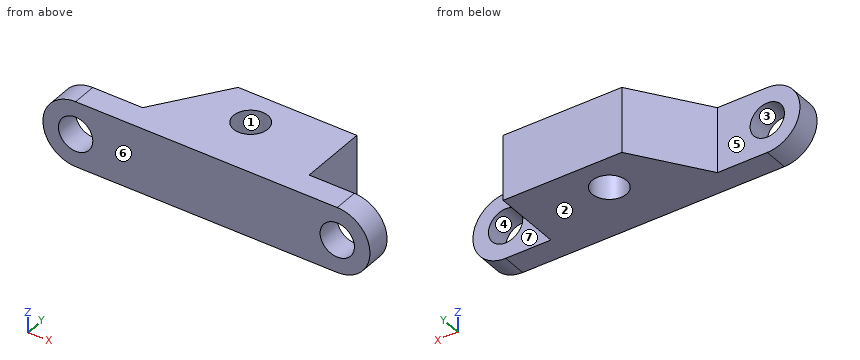
```python
from build123d import *

# Parameters (mm, degrees)
SKETCH1_R           = 2.1
BOSS_EXTRUDE1_DEPTH = 3
SKETCH2_R           = 2.1
BOSS_EXTRUDE2_DEPTH = 8


with BuildPart() as part:
    # Sketch1 → Boss-Extrude1 (new body)
    with BuildSketch(Plane(origin=(0, 0, 0), x_dir=(1, 0, 0), z_dir=(0, 1, 0))):
        with BuildLine():
            Line((0, -4), (32, -4))
            ThreePointArc((32, -4), (36, 0), (32, 4))
            Line((32, 4), (0, 4))
            ThreePointArc((0, 4), (-4, 0), (0, -4))
        make_face()
        with Locations(Location((0, 0, 0), (0, 0, 270))):
            Circle(SKETCH1_R, mode=Mode.SUBTRACT)
        with Locations(Location((32, 0, 0), (0, 0, 270))):
            Circle(SKETCH1_R, mode=Mode.SUBTRACT)
    extrude(amount=BOSS_EXTRUDE1_DEPTH)

    # Sketch2 → Boss-Extrude2 (add)
    with BuildSketch(Plane.XY.offset(4)):
        Polygon((26.470573602, 11.363168568), (11.952968187, 11.363168568), (6.097014513, 3), (20.614619928, 3), (26.470573602, 3), align=None)
        with Locations((16.438382798, 7.127099025)):
            Circle(SKETCH2_R, mode=Mode.SUBTRACT)
    extrude(amount=-BOSS_EXTRUDE2_DEPTH)


solid = part.part
```
Check sheet for the modelled part. Datum: model origin and axes. Units: mm. Face numbers are marked on the shaded views. A direction names the side the tool comes from. Give positions to 0.01 mm unless a question says otherwise; leave off trailing zeros. Write each loop counter-clockwise with the first axis right and the second up, starting at its lowest first coordinate (ties: lowest second). Pieces come first, ordered by that corner, then holes. Notation, with made-up numbers: (4, -28.75) - (29, -28.75) arc R20 ccw to (29, 6.25) - close; hole circle Ø5 at (31, 35). An arc over 180 degrees is marked (long way). Answer as a JSON object with one key per item and string values. Group by question number.
1) Release check for a two-part mould opening along Z. For the marked faces 1, 2, 3 and 4 record: pulls with the +Z half, pulls with the -Z half, needs draft (parallel to the pull), parting line crosses it, or undercut.
2) Sectioned sample at B-B (y = 2.25). Record the cut outline in (x, z).
3) Sectioned sample at D-D (z = 3). Record the cut outline in (x, y), then the cut area to 3 significant figures.
4) Depth check by flat-ended pin: P1, Ø2, axis at y = 9.5, z = 1, coming from the +X side; P2, Ø4, axis at y = 9.5, z = -1.5, coming from the -X side; P3, Ø4, axis at x = 0, z = 0, coming from the +Y side; P4, Ø4, axis at x = 3, z = -2, coming from the +Y side. Enter the tip coordinate at first touch or a pass-through.
5) Sectioned sample at A-A (z = -1.75). Record the cut outline in (x, y), then the cut area to 3 significant figures.
6) Sectioned sample at C-C (y = 7.5). Record the cut outline in (x, z) (3 decimals).
7) Access from +Z, -Z, +X, -X, +Y, -Y to the whole of each face (thin tool, end or side, straight path). Record for the marked faces 5, 6 and 7.
8) Thickness scan on probe 1 along X at (y, z) = (2.3, 0); probe 2 along X at (y, z) = (8.5, -2.75); probe 3 along Y at (x, z) = (4.5, -2). Record the ranges inside material, lowest first. Write a range as from..to.
Geometry results:
{
 "1": {"face 1": "needs draft", "face 2": "pulls with the -Z half", "face 3": "undercut", "face 4": "undercut"},
 "2": {"outline": "(0, -4) - (32, -4) arc R4 ccw to (32, 4) - (0, 4) arc R4 ccw to start; hole circle Ø4.2 at (0, 0); hole circle Ø4.2 at (32, 0)"},
 "3": {"outline": "(-2.65, 0) - (34.65, 0) - (34.65, 3) - (26.47, 3) - (26.47, 11.36) - (11.95, 11.36) - (6.1, 3) - (-2.65, 3) - close; hole circle Ø4.2 at (16.44, 7.13)", "area": "244 mm^2"},
 "4": {"P1": "stops at x = 26.47", "P2": "stops at x = 9.25", "P3": "passes through", "P4": "stops at y = 3"},
 "5": {"outline": "(-3.6, 0) - (-1.16, 0) - (-1.16, 3) - (-3.6, 3) - close; (1.16, 0) - (30.84, 0) - (30.84, 3) - (26.47, 3) - (26.47, 11.36) - (11.95, 11.36) - (6.1, 3) - (1.16, 3) - close; (33.16, 0) - (35.6, 0) - (35.6, 3) - (33.16, 3) - close; hole circle Ø4.2 at (16.44, 7.13)", "area": "236 mm^2"},
 "6": {"outline": "(9.248, -4) - (14.372, -4) - (14.372, 4) - (9.248, 4) - close; (18.505, -4) - (26.471, -4) - (26.471, 4) - (18.505, 4) - close"},
 "7": {"face 5": "+Z, -Z, -X, +Y", "face 6": "+Z, -Z, +X, -X, -Y", "face 7": "+Z, -Z, +X, +Y"},
 "8": {"probe 1": "x = -4..-2.1, 2.1..29.9, 34.1..36", "probe 2": "x = 9.95..14.85, 18.03..26.47", "probe 3": "y = 0..3"}
}
